from build123d import *

# Parameters (mm, degrees)
SKETCH_1_W                   = 90
SKETCH_1_H                   = 73
EXTRUDE_1_DEPTH              = 12
SKETCH_2_R                   = 20
CUT_EXTRUDE_1_DEPTH          = 3
SKETCH_3_R                   = 7.5
CUT_EXTRUDE_2_DEPTH          = 117.232525568
CHAMFER_1_SIZE               = 3
SKETCH_4_W                   = 1
SKETCH_4_H                   = 15
CUT_EXTRUDE_3_DEPTH          = 117.50321884
HOLE_WIZARD_M6_1_D           = 7
HOLE_WIZARD_M6_1_CBORE_D     = 11
HOLE_WIZARD_M6_1_CBORE_DEPTH = 6
HOLE_WIZARD_M5_1_D           = 4.2
HOLE_WIZARD_M5_1_DEPTH       = 12.4
HOLE_WIZARD_M5_1_TIP         = 1.2618073
HOLE_WIZARD_M4_1_D           = 3.3
HOLE_WIZARD_M4_1_DEPTH       = 10.1
HOLE_WIZARD_M4_1_TIP         = 0.991420021
HOLE_WIZARD_M5_2_D           = 4.2
HOLE_WIZARD_M5_2_DEPTH       = 12.4
HOLE_WIZARD_M5_2_TIP         = 1.2618073


with BuildPart() as part:
    # 草图1 → 凸台-拉伸1 (new body)
    with BuildSketch(Plane.XY):
        with Locations((45, 36.5)):
            Rectangle(SKETCH_1_W, SKETCH_1_H)
    extrude(amount=EXTRUDE_1_DEPTH)

    # 草图2 → 切除-拉伸1 (cut)
    with BuildSketch(Plane.XY.offset(12)):
        with Locations((45, 44)):
            Circle(SKETCH_2_R)
    extrude(amount=-CUT_EXTRUDE_1_DEPTH, mode=Mode.SUBTRACT)

    # 草图3 → 切除-拉伸2 (cut, through all)
    with BuildSketch(Plane.XY.offset(9)):
        with Locations((45, 44)):
            Circle(SKETCH_3_R)
    extrude(amount=-CUT_EXTRUDE_2_DEPTH, mode=Mode.SUBTRACT)

    # 倒角1
    chamfer_1_edges = [part.edges().sort_by_distance(p)[0] for p in [
        (0, 73, 6),
        (90, 73, 6),
    ]]
    chamfer(chamfer_1_edges, length=CHAMFER_1_SIZE)

    # 草图4 → 切除-拉伸3 (cut, through all)
    with BuildSketch(Plane(origin=(90, 0, 0), x_dir=(0, 0, -1), z_dir=(1, 0, 0))):
        with Locations((-0.5, 10.5)):
            Rectangle(SKETCH_4_W, SKETCH_4_H)
    extrude(amount=-CUT_EXTRUDE_3_DEPTH, mode=Mode.SUBTRACT)

    # M6 六角凹头螺钉的柱形沉头孔1 (through all)
    with Locations(Plane.XY.offset(12)):
        with Locations((22, 10.5), (68, 10.5)):
            CounterBoreHole(HOLE_WIZARD_M6_1_D / 2, HOLE_WIZARD_M6_1_CBORE_D / 2, HOLE_WIZARD_M6_1_CBORE_DEPTH)

    # M5 螺纹孔1
    with Locations(Plane(origin=(0, 73, 0), x_dir=(-1, 0, 0), z_dir=(0, 1, 0))):
        with Locations((-12, 6), (-78, 6)):
            Hole(HOLE_WIZARD_M5_1_D / 2, depth=HOLE_WIZARD_M5_1_DEPTH)
            with Locations((0, 0, -(HOLE_WIZARD_M5_1_DEPTH + HOLE_WIZARD_M5_1_TIP / 2))):  # 118° drill point
                Cone(0, HOLE_WIZARD_M5_1_D / 2, HOLE_WIZARD_M5_1_TIP, mode=Mode.SUBTRACT)

    # M4 螺纹孔1
    with Locations(Plane.XY.offset(12)):
        with Locations((68.5, 67.5), (21.45, 67.55), (21.45, 20.45), (68.55, 20.45)):
            Hole(HOLE_WIZARD_M4_1_D / 2, depth=HOLE_WIZARD_M4_1_DEPTH)
            with Locations((0, 0, -(HOLE_WIZARD_M4_1_DEPTH + HOLE_WIZARD_M4_1_TIP / 2))):  # 118° drill point
                Cone(0, HOLE_WIZARD_M4_1_D / 2, HOLE_WIZARD_M4_1_TIP, mode=Mode.SUBTRACT)

    # M5 螺纹孔2
    with Locations(Plane.ZY):
        with Locations((6, 43)):
            Hole(HOLE_WIZARD_M5_2_D / 2, depth=HOLE_WIZARD_M5_2_DEPTH)
            with Locations((0, 0, -(HOLE_WIZARD_M5_2_DEPTH + HOLE_WIZARD_M5_2_TIP / 2))):  # 118° drill point
                Cone(0, HOLE_WIZARD_M5_2_D / 2, HOLE_WIZARD_M5_2_TIP, mode=Mode.SUBTRACT)


solid = part.part
Can you work these out from the model? Positions are in its coordinate system, mm. A direction names the side the tool comes from. Give positions to 0.01 mm unless a question says otherwise; leave off trailing zeros. Order: outer loops, then holes, each group sorted by start corner. A loop starts at its lowest first (then second) coordinate and runs counter-clockwise, first axis right, second up. Notation, with made-up numbers: M 73.5,13 L 124.5,13 A22 ccw 124.5,45 Z; hole C 82,60 d4. An arc over 180 degrees is marked long. Use one line per item in the form item = value. Start each with the question number.
Item 1: If I drill on line 1 along X through (y, z) = (20.45, 8); line 2 along X through (y, z) = (67.5, 2.5); line 3 along Y through (x, z) = (68, 8), over which ranges is the centre line in solid material (lowest first)?
Item 2: For faces 5 (the flat face through (46, 10, 1)), 6 (the cylindrical face through (10.452, 66.713, 7.419)), 7 (the flat face through (44, 52, 0)), 8 (the cylindrical face through (64.076, 50.007, 10.521)), which set-ups out of +Z, -Z, +X, -X, +Y, -Y let a thin tool reach every point of the face, with its end or its side?
Item 3: If we section it at A-A (z = 11): Write out the boundary of the cut face in (x, y), then the cut area to 3 significant figures.
Item 4: If we section it at B-B (x = 43): Write out the boundary of the cut face in (y, z).
Item 5: If we section it at C-C (y = 26): Write out the boundary of the cut face in (x, z), then the cut area to 3 significant figures.
Item 6: We'd pull the mould along X, two halves only. Please class faces 1 (the flat face through (44, 2, 0)), 2 (the cylindrical face through (62.505, 10.742, 9.042)), 3 (the cylindrical face through (68.9, 65.9, 6.9)), 4 (the flat face through (90, 35, 6)): +X half, -X half, draft (parallel to the pull), parting line (faces both ways), or undercut.
Item 7: Will these pins go through, and if not, where does the flat tip stop? pin 1 Ø2 at (x, y) = (21.45, 67.55) entering from +Z; pin 2 Ø9 at (x, y) = (68, 10.5) entering from +Z; pin 3 Ø3 at (x, y) = (68.5, 67.5) entering from +Z.
Outcome:
q1.line_1 = 0 to 19.8, 23.1 to 66.9, 70.2 to 90
q1.line_2 = 0 to 19.8, 23.1 to 66.85, 70.15 to 90
q1.line_3 = 0 to 5, 16 to 18.89, 22.01 to 65.93, 69.07 to 73
q2.face_5 = -Z, +X, -X
q2.face_6 = +Y
q2.face_7 = -Z, +X, -X, +Y, -Y
q2.face_8 = +Z
q3.outline = M 0,0 L 90,0 L 90,70 L 87,73 L 3,73 L 0,70 Z; hole C 22,10.5 d11; hole C 21.45,20.45 d3.3; hole C 21.45,67.55 d3.3; hole C 45,44 d40; hole C 68,10.5 d11; hole C 68.5,67.5 d3.3; hole C 68.55,20.45 d3.3
q3.area = 5,080 mm2
q4.outline = M 0,0 L 3,0 L 3,1 L 18,1 L 18,0 L 36.77,0 L 36.77,9 L 24.1,9 L 24.1,12 L 0,12 Z; M 51.23,0 L 73,0 L 73,12 L 63.9,12 L 63.9,9 L 51.23,9 Z
q5.outline = M 0,0 L 90,0 L 90,12 L 53.72,12 L 53.72,9 L 36.28,9 L 36.28,12 L 0,12 Z
q5.area = 1,030 mm2
q6.face_1 = draft
q6.face_2 = undercut
q6.face_3 = undercut
q6.face_4 = +X half
q7.pin_1 = 1.51
q7.pin_2 = 6
q7.pin_3 = 1.81
